For this review, use the dimensioned drawing (mm, ordinates from the lowest corner) and the shaded views. A direction names the side the tool comes from. Round coordinates to 2 decimals unless told otherwise and drop trailing zeros. Write each loop counter-clockwise with the first axis right and the second up, starting at its lowest first coordinate (ties: lowest second). Pieces come first, ordered by that corner, then holes. Notation, with made-up numbers: (7, -1.75) -> (47, -1.75) arc R27 cw to (47, 34.25) -> close; hole circle Ø8 at (15.25, 12). An arc over 180 degrees is marked (long way). Write each question's results on one line, items separated by ' | '. Start each with the question number.
Item 1: Add section B-B (x = 23). State the section outline as (y, z) points.
Item 2: The part is to be moulded in two halves that separate along X. For the marked faces 1, 2 and 3, say which applies: +X half, -X half, draft (parallel to the pull), parting line (faces both ways), or undercut.
Item 3: Clearance check with flat-ended pins moving along their axes: pin 1 (8 mm diameter, centred on y = 15.5, z = 49, fed in from -X); pin 2 (12.5 mm diameter, centred on x = 13.5, y = 13, fed in from +Z); pin 3 (1 mm diameter, centred on x = 28, z = 138.5, fed in from -Y). State where each tip first meets the part, or that it passes through.
Item 4: Tool access review of the marked faces 4, 5 and 6: name each direction out of +Z, -Z, +X, -X, +Y, -Y from which nothing blocks a thin tool from reaching the whole face with its end or side.
Item 5: To check wall thickness, follow line 1 along Z through (x, y) = (27, 19.5); line 2 along Z through (x, y) = (10.5, 20); line 3 along X through (y, z) = (4.5, 185.5). State the ranges of each line that lie inside material, in increasing order.
Item 6: Add section C-C (y = 12.5). State the section outline as (x, z) points, plus the area to 3 significant figures.
Item 7: Add section A-A (z = 176). State the section outline as (x, y) points, plus the area to 4 significant figures.
Item 8: Add section D-D (z = 143). State the section outline as (x, y) points, plus the area to 3 significant figures.
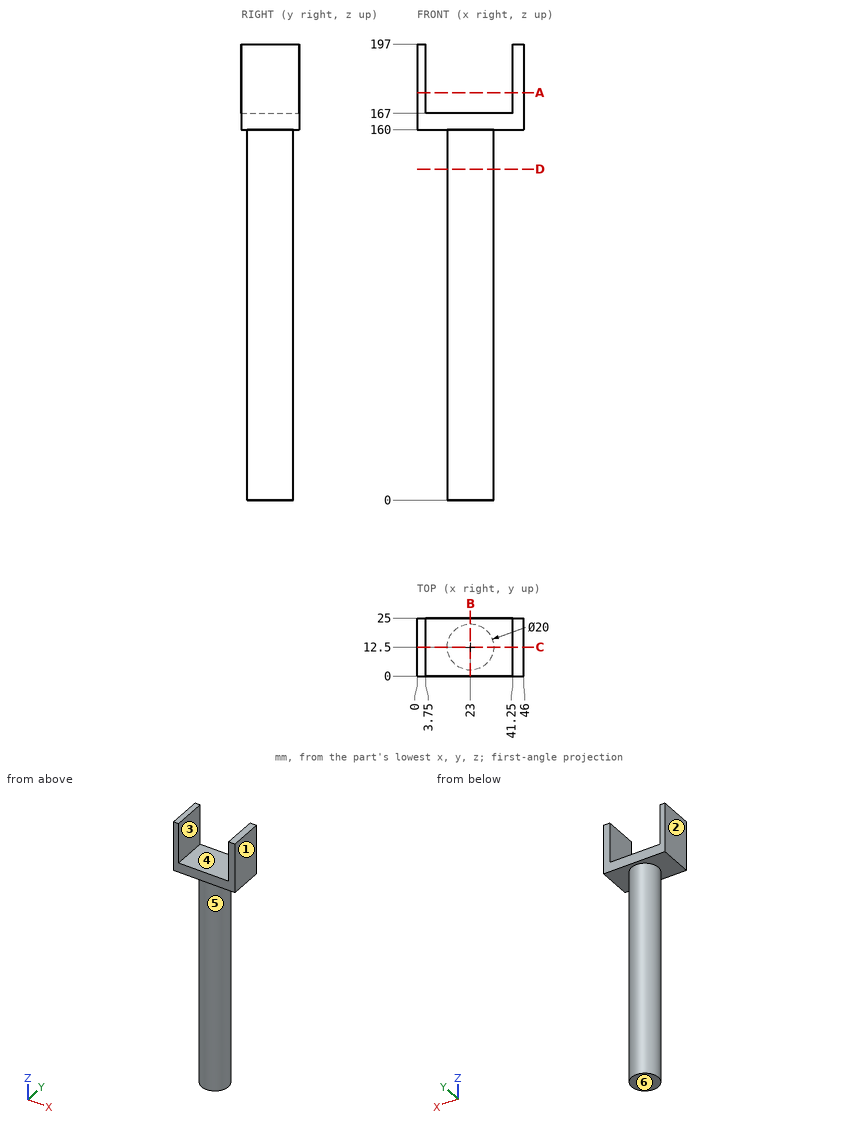
Responses:
1) outline: (0, 160) -> (2.5, 160) -> (2.5, 0) -> (22.5, 0) -> (22.5, 160) -> (25, 160) -> (25, 167) -> (0, 167) -> close
2) face 1: +X half | face 2: -X half | face 3: undercut
3) pin 1: stops at x = 13 | pin 2: stops at z = 167 | pin 3: stops at y = 3.57
4) face 4: +Z, +Y, -Y | face 5: -Z | face 6: -Z, +X, -X, +Y, -Y
5) line 1: z = 0 to 167 | line 2: z = 160 to 167 | line 3: x = 0 to 3.75, 41.25 to 46
6) outline: (0, 160) -> (13, 160) -> (13, 0) -> (33, 0) -> (33, 160) -> (46, 160) -> (46, 197) -> (41.25, 197) -> (41.25, 167) -> (3.75, 167) -> (3.75, 197) -> (0, 197) -> close | area: 3,780 mm^2
7) outline: (0, 0) -> (3.75, 0) -> (3.75, 25) -> (0, 25) -> close; (41.25, 0) -> (46, 0) -> (46, 25) -> (41.25, 25) -> close | area: 212.5 mm^2
8) outline: circle Ø20 at (23, 12.5) | area: 314 mm^2
